Autodesk Inventor part; units mm, degrees
ref_plane "Start Plane" through (0, 0, -4.1685) normal (0, 0, 1) x (1, 0, 0)
ref_plane "End Plane" through (0, 0, 105.9582) normal (0, 0, 1) x (1, 0, 0)
ref_plane "Work Plane4" through (0, 9.525, 105.9582) normal (0, -0.5, 0.866) x (1, 0, 0)
ref_plane "Start Plane" through (0, 0, -4.1685) normal (0, 0, 1) x (1, 0, 0)
ref_plane "End Plane" through (0, 0, 105.9582) normal (0, 0, 1) x (1, 0, 0)
sketch "Sketch" plane through (0, 0, 0) normal (0, 0, 1) x (1, 0, 0)
  circle A0 centre (0, 0) radius 9.525
  dimension "d0" = 19.05
extrude "Body" add sketch "Sketch" along normal up to surface (110.1267 mm away) from surface at -4.1685
sketch "Sketch2" plane through (0, 0, 0) normal (0, 0, 1) x (1, 0, 0)
  line L0 (0, 0) -> (10, 0)
ref_plane "Work Plane3" through (0, 0, 0) normal (0, -1, 0) x (1, 0, 0)
ref_plane "Work Plane4" through (0, 9.525, 105.9582) normal (0, -0.5, 0.866) x (1, 0, 0)
split "Split1" plane through (0, 9.525, 105.9582) removes the side toward (0, -0.5, 0.866)
ref_plane "Work Plane5" through (-4.6367, 8.3203, -3.0644) normal (0.1491, -0.2675, -0.9519) x (0.5375, 0.83, -0.1491)
split "Split2" plane through (-4.6367, 8.3203, -3.0644) removes the side toward (0.1491, -0.2675, -0.9519)
sketch "Sketch3" plane through (0, 0, 0) normal (0, -1, 0) x (1, 0, 0)
  line L0 (-2, -4.1685) -> (12, -4.1685)
  line L1 (-2, 105.9582) -> (12, 105.9582)
  dimension "d7" = 110.1267
equation "\"d0\" = Diam"
equation "\"d1\" = G_L"
equation "\"Diam\" = 19.05"
equation "\"G_L\" = 109.02261"
equation "\"G_OFFSET_START\" = 4.16853"
equation "\"G_OFFSET_END\" = 5.49926"
equation "\"d4\" = -G_OFFSET_START"
equation "\"d5\" = G_OFFSET_END + B_L"
equation "\"B_L\" = 100.45895"
properties part number "ANSI/AISC Rolled Steel - 3/4-4.292, RB" material "Steel, Mild"
Input: part model. Units: mm. Frame: model coordinates. Round coordinates to 2 decimals unless told otherwise and drop trailing zeros. Order: outer loops, then holes, each group sorted by start corner. A loop starts at its lowest first (then second) coordinate and runs counter-clockwise, first axis right, second up.
1. Pin query (flat end, axial travel): P1, Ø4, axis at y = 7, z = 44.5, coming from the -X side; P2, Ø3, axis at y = 4, z = 70.5, coming from the -X side; P3, Ø10, axis at x = 3.5, y = 2, coming from the +Z side; P4, Ø2, axis at y = -0.5, z = 32, coming from the -X side (3 decimals). Return the tip coordinate at first contact, or that it passes through.
The answers:
P1: stops at x = -8.11
P2: stops at x = -9.19
P3: stops at z = 104.5
P4: stops at x = -9.525
2. Cut plane B-B, the plane x = -4.25. Output: boundary loops of the cut face in (y, z).
The answers:
outline: (-8.52, 1.73) - (8.52, -3.06) - (8.52, 105.38) - (-8.52, 95.54) - close
3. Cut plane C-C, the plane y = 4.25. Output: boundary loops of the cut face in (x, z).
The answers:
outline: (-8.52, -2.53) - (8.52, 0.14) - (8.52, 102.91) - (-8.52, 102.91) - close
4. Cut plane A-A, the plane z = 66. Output: boundary loops of the cut face in (x, y) (3 decimals), then the cut area to 3 significant figures.
The answers:
outline: circle Ø19.05 at (0, 0)
area: 285 mm2
5. Material intervals for line 1 (X direction, y = -0.5, z = 12); line 2 (X direction, y = -4, z = 15.5); line 3 (Y direction, x = -6.5, z = 25), sorted ascending.
The answers:
line 1: x = -9.51 to 9.51
line 2: x = -8.64 to 8.64
line 3: y = -6.96 to 6.96
6. Cut plane D-D, the plane z = 98.5. Output: boundary loops of the cut face in (x, y) (3 decimals), then the cut area to 3 significant figures.
The answers:
outline: (-8.9, -3.393) - (8.9, -3.393) arc R9.525 ccw (long way) to start
area: 206 mm2
